Build history of the part. All positions in model axes, mm. A direction names the side the tool comes from. Round coordinates to 2 decimals unless told otherwise and drop trailing zeros. Write each loop counter-clockwise with the first axis right and the second up, starting at its lowest first coordinate (ties: lowest second). Pieces come first, ordered by that corner, then holes. Notation, with made-up numbers: (-16, 22.5) -> (5, 22.5) arc R21 ccw to (5, 44.5) -> close; hole circle Ø1 at (52.5, 66.5). An arc over 180 degrees is marked (long way). Answer in a Markdown table with one row per item. Add a question column.
from build123d import *

# Parameters (mm, degrees)
SKETCH2_W                = 210
SKETCH2_H                = 35
BOSS_EXTRUDE1_DEPTH      = 25
SKETCH3_R                = 5.6
CUT_EXTRUDE1_DEPTH       = 213.205678529
CUT_EXTRUDE2_DEPTH       = 22
SKETCH6_W                = 22.496439662
SKETCH6_H                = 9
BOSS_EXTRUDE3_DEPTH      = 38
CUT_EXTRUDE4_DEPTH       = 17.5
SKETCH9_R                = 2
CUT_EXTRUDE5_DEPTH       = 38
SKETCH10_R               = 2
CUT_EXTRUDE6_DEPTH       = 30
SKETCH12_W               = 4.5
SKETCH12_H               = 5.5
CUT_EXTRUDE7_DEPTH       = 46
SKETCH14_W               = 126.950126738
SKETCH14_H               = 15.619509634
CUT_EXTRUDE8_DEPTH       = 40
FILLET1_R                = 10
SKETCH17_W               = 35
SKETCH17_H               = 25
BOSS_EXTRUDE5_DEPTH      = 180
BOSS_EXTRUDE4_DEPTH      = 20
BOSS_EXTRUDE4_DEPTH_BACK = 25
SKETCH18_R               = 3.130352174
CUT_EXTRUDE9_DEPTH       = 10
SKETCH20_R               = 25.25
CUT_EXTRUDE11_DEPTH      = 30


with BuildPart() as part:
    # Sketch2 → Boss-Extrude1 (new body)
    with BuildSketch(Plane(origin=(0, 0, 0), x_dir=(1, 0, 0), z_dir=(0, 1, 0))):
        with Locations((-105, 0)):
            Rectangle(SKETCH2_W, SKETCH2_H)
    extrude(amount=BOSS_EXTRUDE1_DEPTH)

    # Sketch3 → Cut-Extrude1 (cut, through all)
    with BuildSketch(Plane.XZ):
        with Locations(Location((-21, 0, 0), (0, 0, 270))):
            Circle(SKETCH3_R)
    extrude(amount=-CUT_EXTRUDE1_DEPTH, mode=Mode.SUBTRACT)

    # Sketch4 → Cut-Extrude2 (cut)
    with BuildSketch(Plane(origin=(0, 25, 0), x_dir=(1, 0, 0), z_dir=(0, 1, 0))):
        Polygon((-14.9, 3.521836642), (-21, 7.043673284), (-27.1, 3.521836642), (-27.1, -3.521836642), (-21, -7.043673284), (-14.9, -3.521836642), align=None)
    extrude(amount=-CUT_EXTRUDE2_DEPTH, mode=Mode.SUBTRACT)

    # Sketch6 → Boss-Extrude3 (add)
    with BuildSketch(Plane(origin=(0, 0, 0), x_dir=(0, 0, -1), z_dir=(1, 0, 0))):
        with Locations((0.204742288, 20.5)):
            Rectangle(SKETCH6_W, SKETCH6_H)
    extrude(amount=-BOSS_EXTRUDE3_DEPTH)

    # Sketch7 → Cut-Extrude4 (cut)
    with BuildSketch(Plane.XY.offset(17.5)):
        Polygon((-21, 16), (-14.9, 16), (-14.9, 3), (-15.4, 3), (-15.4, 0), (-26.6, 0), (-26.6, 3), (-27.1, 3), (-27.1, 16), align=None)
    extrude(amount=-CUT_EXTRUDE4_DEPTH, mode=Mode.SUBTRACT)

    # Sketch9 → Cut-Extrude5 (cut)
    with BuildSketch(Plane(origin=(0, 25, 0), x_dir=(1, 0, 0), z_dir=(0, 1, 0))):
        with Locations(Location((-21, 0, 0), (0, 0, 270))):
            Circle(SKETCH9_R)
    extrude(amount=-CUT_EXTRUDE5_DEPTH, mode=Mode.SUBTRACT)

    # Sketch10 → Cut-Extrude6 (cut)
    with BuildSketch(Plane.ZY.offset(210)):
        with Locations((7, 19)):
            Circle(SKETCH10_R)
        with Locations((7, 6)):
            Circle(SKETCH10_R)
        with Locations((-7, 6)):
            Circle(SKETCH10_R)
        with Locations((-7, 19)):
            Circle(SKETCH10_R)
    extrude(amount=-CUT_EXTRUDE6_DEPTH, mode=Mode.SUBTRACT)

    # Sketch12 → Cut-Extrude7 (cut)
    with BuildSketch(Plane(origin=(0, 25, 0), x_dir=(1, 0, 0), z_dir=(0, 1, 0))):
        with Locations((-201.75, -6.75)):
            Rectangle(SKETCH12_W, SKETCH12_H)
        with Locations((-201.75, 6.75)):
            Rectangle(SKETCH12_W, SKETCH12_H)
    extrude(amount=-CUT_EXTRUDE7_DEPTH, mode=Mode.SUBTRACT)

    # Sketch14 → Cut-Extrude8 (cut)
    with BuildSketch(Plane(origin=(0, 25, 0), x_dir=(1, 0, 0), z_dir=(0, 1, 0))):
        with Locations((-105, 0)):
            Rectangle(SKETCH14_W, SKETCH14_H)
    extrude(amount=-CUT_EXTRUDE8_DEPTH, mode=Mode.SUBTRACT)

    # Fillet1
    # the kernel refuses this fillet: 10 mm, written as the material it adds along each edge
    with BuildSketch(Plane(origin=(-168.475063369, 25, 7.809754817), x_dir=(0, 0, -1), z_dir=(0, -1, 0)), Plane(origin=(-41.524936631, 25, 7.809754817), x_dir=(-1, 0, 0), z_dir=(0, -1, 0)), Plane(origin=(-41.524936631, 25, -7.809754817), x_dir=(0, 0, 1), z_dir=(0, -1, 0))) as fillet1_piece_1:
        with BuildLine():
            CenterArc((FILLET1_R, FILLET1_R), FILLET1_R, 180, 90)
            Line((0, FILLET1_R), (0, 0))
            Line((0, 0), (FILLET1_R, 0))
        make_face()
    extrude(amount=25)
    with BuildSketch(Plane(origin=(-168.475063369, 25, -7.809754817), x_dir=(0, 0, 1), z_dir=(0, -1, 0))) as fillet1_piece_2:
        with BuildLine():
            CenterArc((FILLET1_R, -FILLET1_R), FILLET1_R, 90, 90)
            Line((0, -FILLET1_R), (0, 0))
            Line((0, 0), (FILLET1_R, 0))
        make_face()
    extrude(amount=25)

    # Sketch17 → Boss-Extrude5 (add)
    with BuildSketch(Plane(origin=(0, 0, 0), x_dir=(0, 0, -1), z_dir=(1, 0, 0))):
        with Locations((0, 12.5)):
            Rectangle(SKETCH17_W, SKETCH17_H)
    extrude(amount=BOSS_EXTRUDE5_DEPTH)

    # Sketch16 → Boss-Extrude4 (add, two sides: drawn at the far end of the back side and taken through both)
    with BuildSketch(Plane(origin=(0, 25, 0), x_dir=(1, 0, 0), z_dir=(0, 1, 0)).offset(-BOSS_EXTRUDE4_DEPTH_BACK)):
        with BuildLine():
            Line((213.231687746, 28.484303782), (180, 17.5))
            Line((180, 17.5), (180, -17.5))
            Line((180, -17.5), (213.231687746, -28.484303782))
            ThreePointArc((213.231687746, -28.484303782), (252.646805273, 0), (213.231687746, 28.484303782))
        make_face()
    extrude(amount=BOSS_EXTRUDE4_DEPTH + BOSS_EXTRUDE4_DEPTH_BACK)

    # Sketch18 → Cut-Extrude9 (cut)
    with BuildSketch(Plane.ZY.offset(210)):
        with Locations((0, 12.5)):
            Circle(SKETCH18_R)
    extrude(amount=-CUT_EXTRUDE9_DEPTH, mode=Mode.SUBTRACT)

    # Sketch20 → Cut-Extrude11 (cut)
    with BuildSketch(Plane(origin=(0, 45, 0), x_dir=(1, 0, 0), z_dir=(0, 1, 0))):
        with Locations(Location((222.646805273, 0, 0), (0, 0, 270))):
            Circle(SKETCH20_R)
    extrude(amount=-CUT_EXTRUDE11_DEPTH, mode=Mode.SUBTRACT)


solid = part.part
(1) Which spindle directions (+Z, -Z, +X, -X, +Y, -Y) get a long thin tool onto all of the face, cutting with end or side? Do faces 5 (the face through (247.68, 30.21, -3.29)), 6 (the face through (180, 35, 0)), 7 (the face through (-18, 18, 17.5)), 8 (the face through (-27.1, 9, 7)), 9 (the face through (-45.35, 12.675, -5.676)). Say none if no direction does.
(2) Probe line 1 along X through (y, z) = (20, 0); line 2 along Y through (x, z) = (-194, -7); line 3 along Y through (x, z) = (-203.5, 0). List the from-to ranges inside material, lowest first.
(3) Saw through at B-B (y = 36.5). List the corners of the cut face in (x, z), plus the area to 3 significant figures.
(4) Saw through at A-A (x = -66.5). List the corners of the cut face in (y, z), plus the area to 3 significant figures.
(5) Drop flat-ended pins along their axis: P1, Ø8, axis at x = -144, z = 12.5, coming from the +Y side; P2, Ø5, axis at x = -202, y = 18.5, coming from the -Z side; P3, Ø3, axis at y = 19, z = 7, coming from the +X side. Give the stop position or say it passes through.
(6) Mould opens along X. For faces 1 (the face through (-164.797, 12.675, -5.557)), 2 (the face through (196.383, 22.185, 22.915)), 3 (the face through (223, 15, 0)), 4 (the face through (200, 45, 13)) say: pulls with the +X half, pulls with the -X half, needs draft (parallel to the pull), parting line crosses it, or undercut.
(7) Saw through at C-C (x = 149). List the corners of the cut face in (y, z), plus the area to 3 significant figures.
Answer sheet:
| question | item | result |
|---|---|---|
| 1 | face 5 | +Y |
| 1 | face 6 | +Z, -Z, -X, +Y |
| 1 | face 7 | +Z, -X, +Y, -Y |
| 1 | face 8 | +Z |
| 1 | face 9 | +Y, -Y |
| 2 | line 1 | x = -210 to -168.23, -41.77 to -23, -19 to 197.4, 247.9 to 252.65 |
| 2 | line 2 | y = 0 to 4, 8 to 17, 21 to 25 |
| 2 | line 3 | y = 0 to 9.37, 15.63 to 25 |
| 3 | outline | (180, -17.5) -> (213.23, -28.48) arc R30 ccw (long way) to (213.23, 28.48) -> (180, 17.5) -> close; hole circle Ø50.5 at (222.65, 0) |
| 3 | area | 1,490 mm² |
| 4 | outline | (0, -17.5) -> (25, -17.5) -> (25, -7.81) -> (0, -7.81) -> close; (0, 7.81) -> (25, 7.81) -> (25, 17.5) -> (0, 17.5) -> close |
| 4 | area | 485 mm² |
| 5 | P1 | stops at y = 25 |
| 5 | P2 | stops at z = -17.5 |
| 5 | P3 | stops at x = 252.14 |
| 6 | face 1 | undercut |
| 6 | face 2 | pulls with the -X half |
| 6 | face 3 | undercut |
| 6 | face 4 | needs draft |
| 7 | outline | (0, -17.5) -> (25, -17.5) -> (25, 17.5) -> (0, 17.5) -> close |
| 7 | area | 875 mm² |
